Here's the drawing with two shaded views (mm, measured from the low corner). I have some questions. A direction names the side the tool comes from. Coordinates: 2 decimals unless noted, no trailing zeros. Write each loop counter-clockwise with the first axis right and the second up, starting at its lowest first coordinate (ties: lowest second). Pieces come first, ordered by that corner, then holes.
Item 1: If we section it at A-A (x = 9.75): Please give me the cut outline in (y, z).
Item 2: I'm going to push flat-ended pins straight in: pin 1 Ø6 at (x, z) = (12, 14) entering from +Y; pin 2 Ø10 at (x, z) = (4.5, 9.5) entering from +Y; pin 3 Ø10 at (x, z) = (5, 7.5) entering from -Y. Where does each tip first touch, or does it pass through?
Item 3: If we section it at B-B (x = 17.5): Please give me the cut outline in (y, z) (1 decimal), then the cut area to 3 significant figures.
Item 4: If we section it at C-C (x = 15.25): Please give me the cut outline in (y, z) (1 decimal).
Item 5: If I drill on line 1 (Y direction, x = 9.75, z = 7.5); line 2 (X direction, y = 1.75, z = 6.75), over which ranges is the centre line in solid material (lowest first)?
Item 6: We'd pull the mould along Z, two halves only. Please class the marked faces 1, 2, 3 and 4: +Z half, -Z half, draft (parallel to the pull), parting line (faces both ways), or undercut.
Item 7: For the marked faces 5, 6, 7 and 8, which set-ups out of +Z, -Z, +X, -X, +Y, -Y let a thin tool reach every point of the face, with its end or its side?
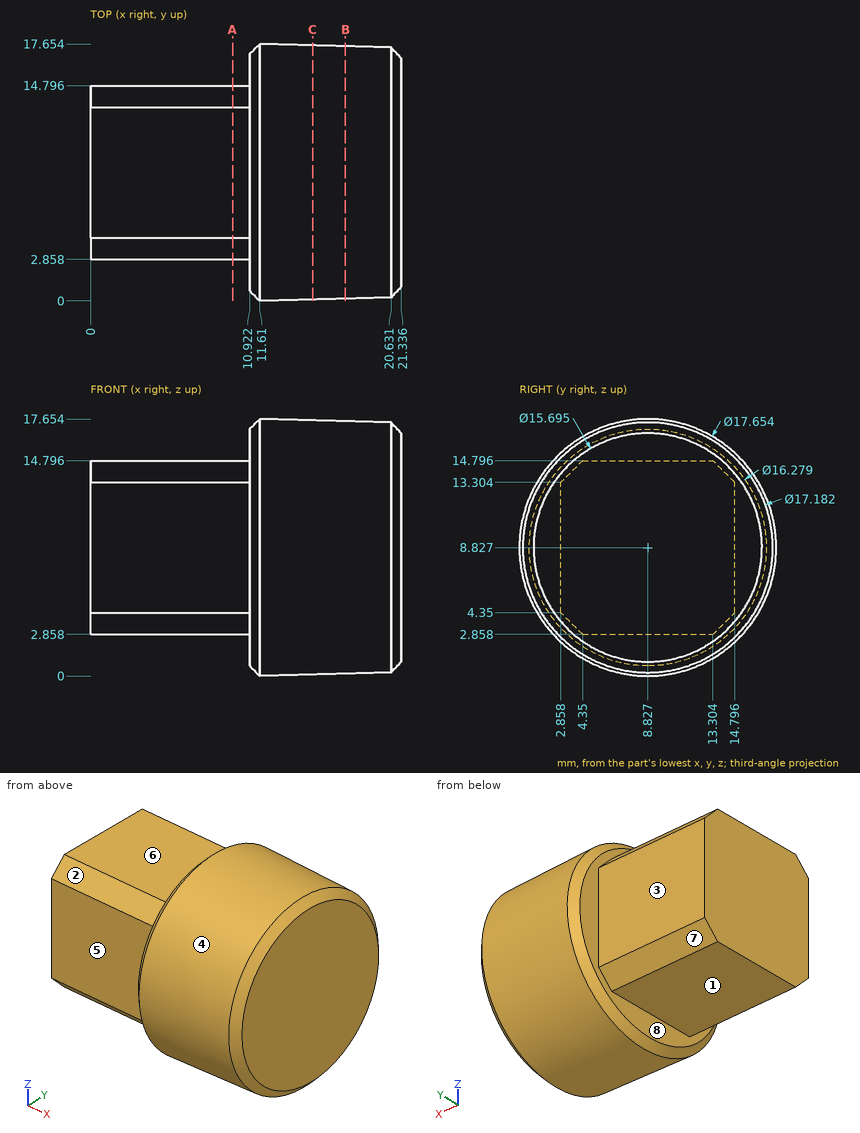
Answer list:
1. outline: (2.86, 4.35) - (4.35, 2.86) - (13.3, 2.86) - (14.8, 4.35) - (14.8, 13.3) - (13.3, 14.8) - (4.35, 14.8) - (2.86, 13.3) - close
2. pin 1: stops at y = 17.38
2. pin 2: stops at y = 14.8
2. pin 3: stops at y = 2.86
3. outline: circle Ø17.3 at (8.8, 8.8)
3. area: 236 mm2
4. outline: circle Ø17.5 at (8.8, 8.8)
5. line 1: y = 2.86 to 14.8
5. line 2: x = 10.92 to 21.34
6. face 1: -Z half
6. face 2: +Z half
6. face 3: draft
6. face 4: parting line
7. face 5: +Z, -Z, -X, -Y
7. face 6: +Z, -X, +Y, -Y
7. face 7: -Z, -X, +Y
7. face 8: -X
